The model under review builds one solid part; all positions refer to its coordinate system, in mm. Round coordinates to 2 decimals unless told otherwise and drop trailing zeros. Order: outer loops, then holes, each group sorted by start corner. A loop starts at its lowest first (then second) coordinate and runs counter-clockwise, first axis right, second up. Notation, with made-up numbers: M 39.5,1.25 L 52.5,1.25 A22 cw 52.5,34.25 Z; hole C 10,89 d9. An arc over 180 degrees is marked long. Answer as a JSON object with one key per item and string values. Group by question number.
1) Insertion check: pin 1 Ø1 at (y, z) = (-1.5, -1) entering from -X. The pin has a flat end and moves straight along its axis. Give the tip position at first contact, or say it passes through.
2) Consider section A-A, the plane x = -8.5. Write out the cut boundary in (y, z).
3) Consider section B-B, the plane y = -2. Count the separate pieces of the cut face and the enclosed holes in it, then the cut area to 3 significant figures.
4) Consider section C-C, the plane z = -32. Write out the cut boundary in (x, y).
5) The part is to be moulded in two halves that separate along Z. For faces 1 (the flat face through (-9.198, -1.377, -27.618)), 2 (the flat face through (-20, 0, -19)), 3 (the cylindrical face through (-21.994, -1.377, 61.602)), say which applies: +Z half, -Z half, draft (parallel to the pull), parting line (faces both ways), or undercut.
6) To check wall thickness, follow line 1 (Z direction, x = -21, y = -2.3); line 2 (Z direction, x = -23, y = -2.45); line 3 (Z direction, x = 23.5, y = -0.45). State the ranges of each line that lie inside material, in increasing order.
7) Consider section D-D, the plane x = -33. Write out the cut boundary in (y, z).
```python
from build123d import *

# Parameters (mm, degrees)
F0_R     = 3.175
F1_DEPTH = 2.794


with BuildPart() as f1:
    # F0 (on Front) → F1 (new body)
    with BuildSketch(Plane.XZ):
        with BuildLine():
            Line((-37.5902472441, 5.1871481091), (-38.0787087825, 1.2794558015))
            ThreePointArc((-38.0787087825, 1.2794558015), (-38.0378492862, 0.1412029688), (-37.9154811276, -0.9911905332))
            ThreePointArc((-37.9154811276, -0.9911905332), (-32.5952706102, -10.7218386196), (-22.2037087825, -14.5955441985))
            Line((-22.2037087825, -14.5955441985), (-22.2037087825, -1.8955441985))
            ThreePointArc((-22.2037087825, -1.8955441985), (-25.3787087825, 1.2794558015), (-22.2037087825, 4.4544558015))
            Line((-22.2037087825, 4.4544558015), (-22.2037087825, 17.1544558015))
            ThreePointArc((-22.2037087825, 17.1544558015), (-31.9500160221, 13.8104222523), (-37.5902472441, 5.1871481091))
        make_face()
        with BuildLine():
            ThreePointArc((-37.5902472441, 5.1871481091), (-37.9561200754, 3.2485072131), (-38.0787087825, 1.2794558015))
            Line((-38.0787087825, 1.2794558015), (-37.5902472441, 5.1871481091))
        make_face()
        with BuildLine():
            ThreePointArc((-22.2037087825, -14.5955441985), (-32.5952706102, -10.7218386196), (-37.9154811276, -0.9911905332))
            Line((-37.9154811276, -0.9911905332), (-31.7287087825, -62.2205441985))
            ThreePointArc((-31.7287087825, -62.2205441985), (-28.9389008733, -55.4853521077), (-22.2037087825, -52.6955441985))
            Line((-22.2037087825, -52.6955441985), (-22.2037087825, -14.5955441985))
        make_face()
        with BuildLine():
            Line((-31.7287087825, 52.0794558015), (-37.5902472441, 5.1871481091))
            ThreePointArc((-37.5902472441, 5.1871481091), (-31.9500160221, 13.8104222523), (-22.2037087825, 17.1544558015))
            Line((-22.2037087825, 17.1544558015), (-22.2037087825, 38.2629670203))
            Line((-22.2037087825, 38.2629670203), (-22.2037087825, 42.5544558015))
            ThreePointArc((-22.2037087825, 42.5544558015), (-28.9389008733, 45.3442637107), (-31.7287087825, 52.0794558015))
        make_face()
        with Locations((-25.8746817708, 38.2629670203)):
            Circle(F0_R, mode=Mode.SUBTRACT)
        with BuildLine():
            Line((-22.2037087825, -1.8955441985), (-22.2037087825, -14.5955441985))
            ThreePointArc((-22.2037087825, -14.5955441985), (-11.9871413621, -10.871156329), (-6.5643326528, -1.4455284687))
            ThreePointArc((-6.5643326528, -1.4455284687), (-6.3877244461, -0.0881203281), (-6.3287087825, 1.2794558015))
            Line((-6.3287087825, 1.2794558015), (-6.817170321, 5.1871481091))
            ThreePointArc((-6.817170321, 5.1871481091), (-12.457401543, 13.8104222523), (-22.2037087825, 17.1544558015))
            Line((-22.2037087825, 17.1544558015), (-22.2037087825, 4.4544558015))
            ThreePointArc((-22.2037087825, 4.4544558015), (-19.9586447523, 3.5245198317), (-19.0287087825, 1.2794558015))
            ThreePointArc((-19.0287087825, 1.2794558015), (-19.9586447523, -0.9656082288), (-22.2037087825, -1.8955441985))
        make_face()
        with BuildLine():
            ThreePointArc((-6.5643326528, -1.4455284687), (-11.9871413621, -10.871156329), (-22.2037087825, -14.5955441985))
            Line((-22.2037087825, -14.5955441985), (-22.2037087825, -52.6955441985))
            ThreePointArc((-22.2037087825, -52.6955441985), (-21.8637469544, -52.7016130109), (-21.5242183367, -52.7198117145))
            Line((-21.5242183367, -52.7198117145), (-11.7579621852, -53.068606577))
            Line((-11.7579621852, -53.068606577), (-6.5643326528, -1.4455284687))
        make_face()
        with BuildLine():
            ThreePointArc((-22.2037087825, -52.6955441985), (-28.9389008733, -55.4853521077), (-31.7287087825, -62.2205441985))
            ThreePointArc((-31.7287087825, -62.2205441985), (-28.9389008733, -68.9557362893), (-22.2037087825, -71.7455441985))
            Line((-22.2037087825, -71.7455441985), (-21.5242183367, -71.7212766826))
            ThreePointArc((-21.5242183367, -71.7212766826), (-15.2324186761, -68.711055677), (-12.6787087825, -62.2205441985))
            Line((-12.6787087825, -62.2205441985), (-19.0287087825, -62.2205441985))
            ThreePointArc((-19.0287087825, -62.2205441985), (-24.4487728128, -64.4656082288), (-22.2037087825, -59.0455441985))
            Line((-22.2037087825, -59.0455441985), (-22.2037087825, -52.6955441985))
        make_face()
        with BuildLine():
            Line((-22.2037087825, 38.2629670203), (-22.2037087825, 17.1544558015))
            ThreePointArc((-22.2037087825, 17.1544558015), (-12.457401543, 13.8104222523), (-6.817170321, 5.1871481091))
            Line((-6.817170321, 5.1871481091), (-12.6787087825, 52.0794558015))
            ThreePointArc((-12.6787087825, 52.0794558015), (-15.4685166917, 45.3442637107), (-22.2037087825, 42.5544558015))
            Line((-22.2037087825, 42.5544558015), (-22.2037087825, 38.2629670203))
        make_face()
        with BuildLine():
            ThreePointArc((-12.6787087825, 52.0794558015), (-22.2037087825, 61.6044558015), (-31.7287087825, 52.0794558015))
            ThreePointArc((-31.7287087825, 52.0794558015), (-28.9389008733, 45.3442637107), (-22.2037087825, 42.5544558015))
            ThreePointArc((-22.2037087825, 42.5544558015), (-15.4685166917, 45.3442637107), (-12.6787087825, 52.0794558015))
        make_face()
        with BuildLine():
            ThreePointArc((-19.0287087825, 52.0794558015), (-19.9586447523, 49.8343917712), (-22.2037087825, 48.9044558015))
            ThreePointArc((-22.2037087825, 48.9044558015), (-24.4487728128, 54.3245198317), (-19.0287087825, 52.0794558015))
        make_face(mode=Mode.SUBTRACT)
        with BuildLine():
            Line((-21.5242183367, -71.7212766826), (-22.2037087825, -71.7455441985))
            ThreePointArc((-22.2037087825, -71.7455441985), (-21.8637469544, -71.7394753862), (-21.5242183367, -71.7212766826))
        make_face()
        with BuildLine():
            ThreePointArc((-6.3287087825, 1.2794558015), (-6.4512974897, 3.2485072131), (-6.817170321, 5.1871481091))
            Line((-6.817170321, 5.1871481091), (-6.3287087825, 1.2794558015))
        make_face()
        with BuildLine():
            Line((22.2462912175, -54.2830441985), (-11.7579621852, -53.068606577))
            Line((-11.7579621852, -53.068606577), (-12.6787087825, -62.2205441985))
            Line((-12.6787087825, -62.2205441985), (14.3087912175, -62.2205441985))
            ThreePointArc((14.3087912175, -62.2205441985), (16.6336311418, -56.6078841229), (22.2462912175, -54.2830441985))
        make_face()
        with BuildLine():
            Line((-12.6787087825, -62.2205441985), (-11.7579621852, -53.068606577))
            Line((-11.7579621852, -53.068606577), (-21.5242183367, -52.7198117145))
            ThreePointArc((-21.5242183367, -52.7198117145), (-15.2324186761, -55.7300327201), (-12.6787087825, -62.2205441985))
        make_face()
        with BuildLine():
            ThreePointArc((-12.6787087825, -62.2205441985), (-15.2324186761, -68.711055677), (-21.5242183367, -71.7212766826))
            Line((-21.5242183367, -71.7212766826), (22.2462912175, -70.1580441985))
            ThreePointArc((22.2462912175, -70.1580441985), (16.6336311418, -67.8332042742), (14.3087912175, -62.2205441985))
            Line((14.3087912175, -62.2205441985), (-12.6787087825, -62.2205441985))
        make_face()
        with BuildLine():
            ThreePointArc((30.1837912175, -62.2205441985), (27.8589512931, -56.6078841229), (22.2462912175, -54.2830441985))
            ThreePointArc((22.2462912175, -54.2830441985), (16.6336311418, -56.6078841229), (14.3087912175, -62.2205441985))
            ThreePointArc((14.3087912175, -62.2205441985), (16.6336311418, -67.8332042742), (22.2462912175, -70.1580441985))
            ThreePointArc((22.2462912175, -70.1580441985), (27.8589512931, -67.8332042742), (30.1837912175, -62.2205441985))
        make_face()
        with BuildLine():
            ThreePointArc((25.4212912175, -62.2205441985), (22.2462912175, -65.3955441985), (19.0712912175, -62.2205441985))
            ThreePointArc((19.0712912175, -62.2205441985), (22.2462912175, -59.0455441985), (25.4212912175, -62.2205441985))
        make_face(mode=Mode.SUBTRACT)
        with BuildLine():
            Line((-21.5242183367, -52.7198117145), (-22.2037087825, -52.6955441985))
            Line((-22.2037087825, -52.6955441985), (-22.2037087825, -59.0455441985))
            ThreePointArc((-22.2037087825, -59.0455441985), (-19.9586447523, -59.9754801683), (-19.0287087825, -62.2205441985))
            Line((-19.0287087825, -62.2205441985), (-12.6787087825, -62.2205441985))
            ThreePointArc((-12.6787087825, -62.2205441985), (-15.2324186761, -55.7300327201), (-21.5242183367, -52.7198117145))
        make_face()
    extrude(amount=F1_DEPTH)


solid = f1.part
```
Results list:
{
 "1": {"pin 1": "x = -37.98"},
 "2": {"outline": "M -2.79,-71.26 L 0,-71.26 L 0,-53.18 L -2.79,-53.18 Z; M -2.79,-20.69 L 0,-20.69 L 0,18.65 L -2.79,18.65 Z"},
 "3": {"separate pieces": "1", "enclosed holes": "6", "area": "3,740 mm^2"},
 "4": {"outline": "M -34.78,-2.79 L -9.64,-2.79 L -9.64,0 L -34.78,0 Z"},
 "5": {"face 1": "undercut", "face 2": "draft", "face 3": "+Z half"},
 "6": {"line 1": "-71.7 to -65.16, -59.28 to -1.66, 4.22 to 49.14, 55.02 to 61.53", "line 2": "-71.71 to -65.29, -59.15 to -1.79, 4.35 to 36.92, 39.61 to 49.01, 55.15 to 61.57", "line 3": "-70.06 to -65.14, -59.3 to -54.38"},
 "7": {"outline": "M -2.79,-49.64 L 0,-49.64 L 0,41.91 L -2.79,41.91 Z"}
}
